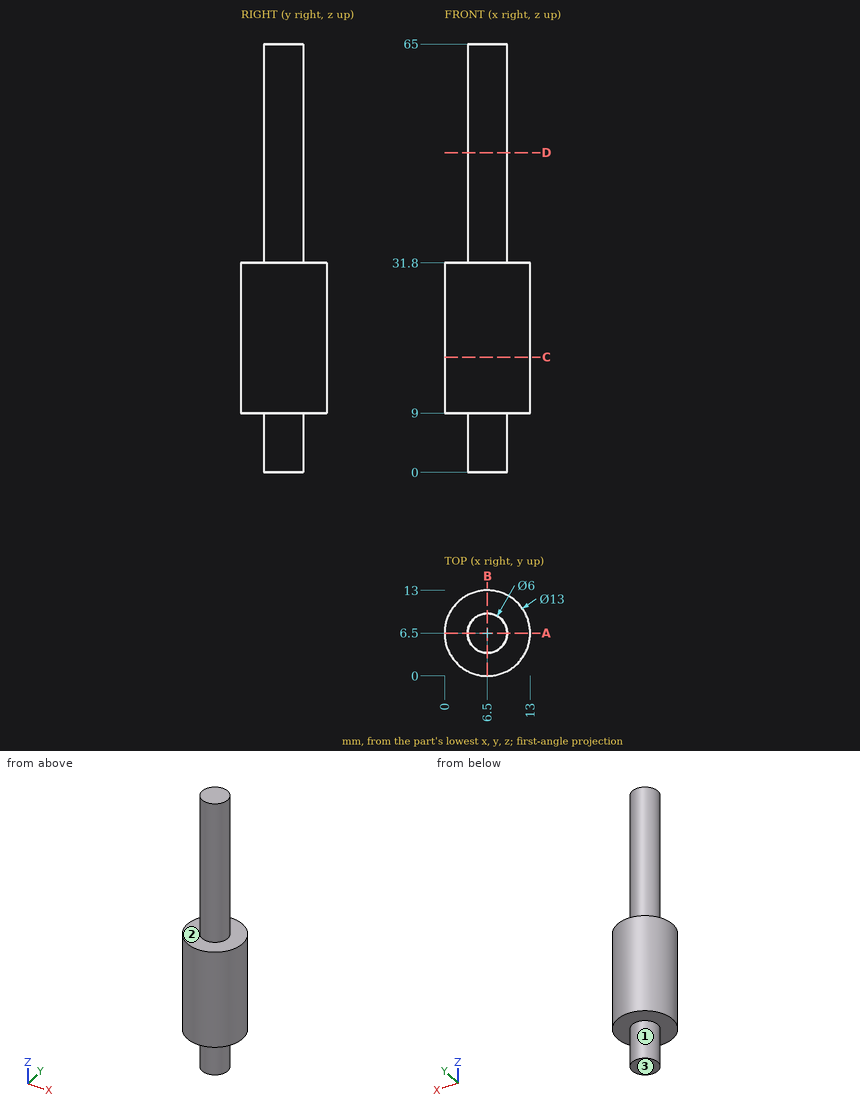
Source: three-view drawing plus pictorial views. Frame: mm from the lowest corner of the part. A direction names the side the tool comes from. Give positions to 0.01 mm unless a question says otherwise; leave off trailing zeros. Write each loop counter-clockwise with the first axis right and the second up, starting at its lowest first coordinate (ties: lowest second). Pieces come first, ordered by that corner, then holes.
(1) Cut plane D-D, the plane z = 48.5. Return loops of the section in (x, y), then the cut area to 3 significant figures.
(2) Cut plane A-A, the plane y = 6.5. Return loops of the section in (x, z).
(3) Cut plane C-C, the plane z = 17.5. Return loops of the section in (x, y).
(4) Access query for the marked faces 1, 2 and 3. Directions: +Z, -Z, +X, -X, +Y, -Y. A direction counts if a zero-diameter tool reaches every point of the face in a straight line with its end or side. Return the directions, or none.
(5) Ray query, line 1 (Z direction, x = 11.5, y = 10.25); line 2 (Y direction, x = 6.5, z = 5); line 3 (Y direction, x = 5.25, z = 34). Return the intervals inside material, ascending.
(6) First-contact query: P1, Ø5, axis at y = 9, z = 45.5, coming from the -X side; P2, Ø2, axis at x = 3, y = 9, coming from the +Z side; P3, Ø2, axis at x = 4.5, z = 16.5, coming from the -Y side. Flat tips, straight axial feed; report the tip coordinate or a pass-through.
Values follow:
1. outline: circle Ø6 at (6.5, 6.5)
1. area: 28.3 mm2
2. outline: (0, 9) - (3.5, 9) - (3.5, 0) - (9.5, 0) - (9.5, 9) - (13, 9) - (13, 31.8) - (9.5, 31.8) - (9.5, 65) - (3.5, 65) - (3.5, 31.8) - (0, 31.8) - close
3. outline: circle Ø13 at (6.5, 6.5)
4. face 1: -Z
4. face 2: +Z
4. face 3: -Z, +X, -X, +Y, -Y
5. line 1: z = 9 to 31.8
5. line 2: y = 3.5 to 9.5
5. line 3: y = 3.77 to 9.23
6. P1: stops at x = 3.5
6. P2: stops at z = 31.8
6. P3: stops at y = 0.08
